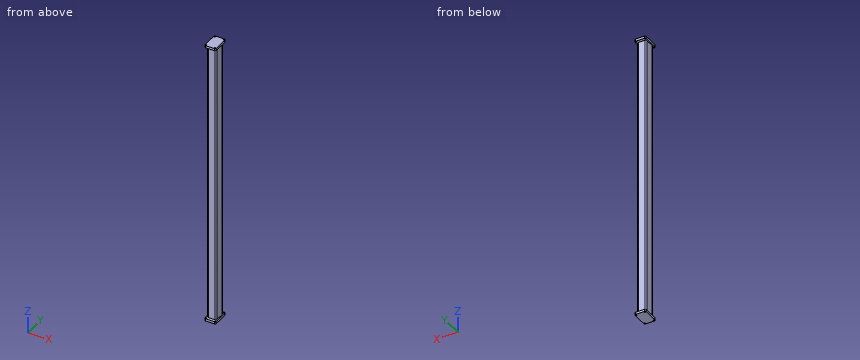
from build123d import *

# Parameters (mm, degrees)
SKETCH_1_R        = 0.5
EXTRUDE_1_DEPTH   = 2
SKETCH_2_W        = 6
SKETCH_2_H        = 8
EXTRUDE_1_2_DEPTH = 126
SCALE_1_SCALE     = 2
SCALE_2_SCALE     = 1.7


with BuildPart() as part:
    # 草图1 → Extrude 1 (new body)
    with BuildSketch(Plane.XY):
        with BuildLine():
            Line((-4, 7.5), (4, 7.5))
            ThreePointArc((4, 7.5), (4.707106781, 7.207106781), (5, 6.5))
            Line((5, 6.5), (5, -6.5))
            ThreePointArc((5, -6.5), (4.707106781, -7.207106781), (4, -7.5))
            Line((4, -7.5), (-4, -7.5))
            ThreePointArc((-4, -7.5), (-4.707106781, -7.207106781), (-5, -6.5))
            Line((-5, -6.5), (-5, 6.5))
            ThreePointArc((-5, 6.5), (-4.707106781, 7.207106781), (-4, 7.5))
        make_face()
        with Locations((4, 6.5)):
            Circle(SKETCH_1_R, mode=Mode.SUBTRACT)
        with Locations((-4, 6.5)):
            Circle(SKETCH_1_R, mode=Mode.SUBTRACT)
        with Locations((4, -6.5)):
            Circle(SKETCH_1_R, mode=Mode.SUBTRACT)
        with Locations((-4, -6.5)):
            Circle(SKETCH_1_R, mode=Mode.SUBTRACT)
    extrude(amount=EXTRUDE_1_DEPTH)

    # 草图2 → Extrude 1 2 (add)
    with BuildSketch(Plane(origin=(0, 0, 0), x_dir=(-1, 0, 0), z_dir=(0, 0, -1))):
        with BuildLine():
            Line((-3, 5), (3, 5))
            ThreePointArc((3, 5), (3.707106781, 4.707106781), (4, 4))
            Line((4, 4), (4, -4))
            ThreePointArc((4, -4), (3.707106781, -4.707106781), (3, -5))
            Line((3, -5), (-3, -5))
            ThreePointArc((-3, -5), (-3.707106781, -4.707106781), (-4, -4))
            Line((-4, -4), (-4, 4))
            ThreePointArc((-4, 4), (-3.707106781, 4.707106781), (-3, 5))
        make_face()
        Rectangle(SKETCH_2_W, SKETCH_2_H, mode=Mode.SUBTRACT)
    extrude(amount=EXTRUDE_1_2_DEPTH)

    # 镜向1: part across plane


with BuildPart() as part_1:
    add(part.part)
    add(part.part.mirror(Plane(origin=(3, -4, -126), x_dir=(1, 0, 0), z_dir=(0, 0, -1))))


with BuildPart() as part_2:
    # 缩放比例1: scaled about (0, 0, 0)
    add(part_1.part.scale(SCALE_1_SCALE))


with BuildPart() as part_3:
    # 缩放比例2: scaled about (0, 0, 0)
    add(part_2.part.scale(SCALE_2_SCALE))


solid = part_3.part
Source: CAD feature listing. Evaluate the final solid. Frame: model axes, mm. Coordinates: 2 decimals unless noted, no trailing zeros. Loops run counter-clockwise (first coordinate to the right, second up) from the corner with the lowest first, then second, coordinate; pieces in that order, holes last. Notation, with made-up numbers: (29, 44) -> (79, 44) arc R23 ccw to (79, 80) -> close; hole circle Ø10 at (-40, 17.5). An arc over 180 degrees is marked (long way). Answer in a Markdown table with one row per item. Add a question column.
Q1. Section A-A on y = -4. Return the cut outline in (x, z).
Q2. Contact query for flat-ended pins moving along their axis: pin 1 Ø10 at (x, z) = (-12, -727.5) entering from -Y; pin 2 Ø6 at (x, z) = (0.5, -597.5) entering from +Y; pin 3 Ø6 at (y, z) = (-2.5, -247) entering from -X. Output: stop coordinate, or through.
Q3. Ray query, line 1 along Y through (x, z) = (13.6, 3.5); line 2 along Y through (x, z) = (13, 4); line 3 along X through (y, z) = (-10.5, -828). Return the intervals inside material, ascending.
Q4. Section C-C on z = -94. Return the cut outline in (x, y).
Q5. Section B-B on x = 5. Return the cut outline in (y, z), and give its area (3 significant figures).
Computed values:
| question | item | result |
|---|---|---|
| 1 | outline | (-17, -863.6) -> (17, -863.6) -> (17, -856.8) -> (13.6, -856.8) -> (13.6, 0) -> (17, 0) -> (17, 6.8) -> (-17, 6.8) -> (-17, 0) -> (-13.6, 0) -> (-13.6, -856.8) -> (-17, -856.8) -> close; hole (-10.2, -856.8) -> (10.2, -856.8) -> (10.2, 0) -> (-10.2, 0) -> close |
| 2 | pin 1 | stops at y = -17 |
| 2 | pin 2 | stops at y = 17 |
| 2 | pin 3 | stops at x = -13.6 |
| 3 | line 1 | y = -25.5 to -23.8, -20.4 to 20.4, 23.8 to 25.5 |
| 3 | line 2 | y = -25.5 to -23.69, -20.51 to 20.51, 23.69 to 25.5 |
| 3 | line 3 | x = -13.6 to -10.2, 10.2 to 13.6 |
| 4 | outline | (-13.6, -13.6) arc R3.4 ccw to (-10.2, -17) -> (10.2, -17) arc R3.4 ccw to (13.6, -13.6) -> (13.6, 13.6) arc R3.4 ccw to (10.2, 17) -> (-10.2, 17) arc R3.4 ccw to (-13.6, 13.6) -> close; hole (-10.2, -13.6) -> (10.2, -13.6) -> (10.2, 13.6) -> (-10.2, 13.6) -> close |
| 5 | outline | (-25.5, -863.6) -> (25.5, -863.6) -> (25.5, -856.8) -> (17, -856.8) -> (17, 0) -> (25.5, 0) -> (25.5, 6.8) -> (-25.5, 6.8) -> (-25.5, 0) -> (-17, 0) -> (-17, -856.8) -> (-25.5, -856.8) -> close; hole (-13.6, -856.8) -> (13.6, -856.8) -> (13.6, 0) -> (-13.6, 0) -> close |
| 5 | area | 6,520 mm^2 |
